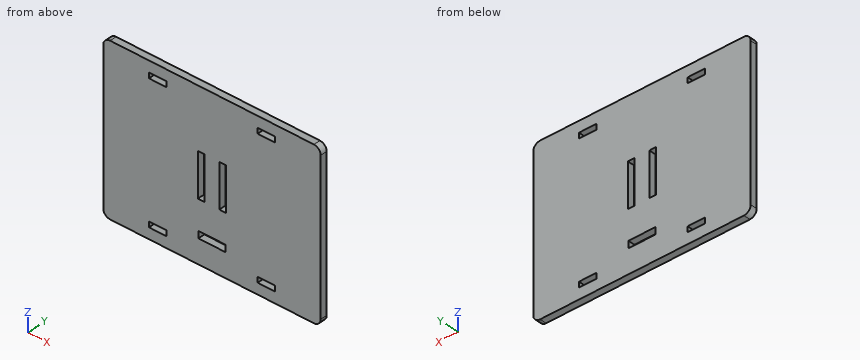
```python
from build123d import *

# Parameters (mm, degrees)
SKETCH1_W           = 101.6
SKETCH1_H           = 76.2
SKETCH1_W_2         = 8.128
SKETCH1_H_2         = 2.54
BOSS_EXTRUDE1_DEPTH = 3.175
FILLET1_R           = 3.175
SKETCH2_W           = 3.175
SKETCH2_H           = 20.32
SKETCH2_W_2         = 12.7
SKETCH2_H_2         = 3.2004
CUT_EXTRUDE1_DEPTH  = 3.175


with BuildPart() as part:
    # Sketch1 → Boss-Extrude1 (new body)
    with BuildSketch(Plane(origin=(0, 0, 0), x_dir=(1, 0, 0), z_dir=(0, 1, 0))):
        Rectangle(SKETCH1_W, SKETCH1_H)
        with Locations((-25.4, 31.75)):
            Rectangle(SKETCH1_W_2, SKETCH1_H_2, mode=Mode.SUBTRACT)
        with Locations((-25.4, -31.75)):
            Rectangle(SKETCH1_W_2, SKETCH1_H_2, mode=Mode.SUBTRACT)
        with Locations((25.4, -31.75)):
            Rectangle(SKETCH1_W_2, SKETCH1_H_2, mode=Mode.SUBTRACT)
        with Locations((25.4, 31.75)):
            Rectangle(SKETCH1_W_2, SKETCH1_H_2, mode=Mode.SUBTRACT)
    extrude(amount=BOSS_EXTRUDE1_DEPTH)

    # Fillet1
    fillet1_edges = [part.edges().sort_by_distance(p)[0] for p in [
        (50.8, 1.5875, 38.1),
        (-50.8, 1.5875, 38.1),
        (-50.8, 1.5875, -38.1),
        (50.8, 1.5875, -38.1),
    ]]
    fillet(fillet1_edges, radius=FILLET1_R)

    # Sketch2 → Cut-Extrude1 (cut)
    with BuildSketch(Plane(origin=(0, 3.175, 0), x_dir=(1, 0, 0), z_dir=(0, 1, 0))):
        with Locations((-5.0165, 0)):
            Rectangle(SKETCH2_W, SKETCH2_H)
        with Locations((5.0165, 0)):
            Rectangle(SKETCH2_W, SKETCH2_H)
        with Locations((0, 25.4)):
            Rectangle(SKETCH2_W_2, SKETCH2_H_2)
    extrude(amount=-CUT_EXTRUDE1_DEPTH, mode=Mode.SUBTRACT)


solid = part.part
```
Design review of the part built by this model. Coordinates are the model's own, in mm. Give positions to 0.01 mm unless a question says otherwise; leave off trailing zeros. Write each loop counter-clockwise with the first axis right and the second up, starting at its lowest first coordinate (ties: lowest second). Pieces come first, ordered by that corner, then holes.
(1) Clearance check with a flat-ended pin moving along its axis: pin 1 Ø1.5 at (x, z) = (5, -3) entering from +Y. State where the tip first meets the part, or that it passes through.
Checked values:
pin 1: passes through
(2) Add section A-A (x = 24.5). Give the boundary of the cut face in (y, z) (3 decimals).
Checked values:
outline: (0, -38.1) - (3.175, -38.1) - (3.175, -33.02) - (0, -33.02) - close; (0, -30.48) - (3.175, -30.48) - (3.175, 30.48) - (0, 30.48) - close; (0, 33.02) - (3.175, 33.02) - (3.175, 38.1) - (0, 38.1) - close
(3) Add section C-C (y = 2.35). Give the number of separate pieces and of enclosed holes in the cut face, and give its area (3 significant figures).
Checked values:
separate pieces: 1
enclosed holes: 7
area: 7,480 mm2
(4) Add section B-B (z = -7.5). Give the boundary of the cut face in (x, y) (3 decimals), and give its area (3 significant figures).
Checked values:
outline: (-50.8, 0) - (-6.604, 0) - (-6.604, 3.175) - (-50.8, 3.175) - close; (-3.429, 0) - (3.429, 0) - (3.429, 3.175) - (-3.429, 3.175) - close; (6.604, 0) - (50.8, 0) - (50.8, 3.175) - (6.604, 3.175) - close
area: 302 mm2
(5) Wall thickness on line 1 along X through (y, z) = (2.6, -3); line 2 along Z through (x, y) = (-24, 0.65); line 3 along Z through (x, y) = (3, 2.85): over which ranges is each line inside the solid? List them lowest first.
Checked values:
line 1: x = -50.8 to -6.6, -3.43 to 3.43, 6.6 to 50.8
line 2: z = -38.1 to -33.02, -30.48 to 30.48, 33.02 to 38.1
line 3: z = -38.1 to -27, -23.8 to 38.1
